Check sheet for the drawn part. Datum: minimum x, y, z corner. Units: mm. A direction names the side the tool comes from. Coordinates: 2 decimals unless noted, no trailing zeros. Order: outer loops, then holes, each group sorted by start corner. A loop starts at its lowest first (then second) coordinate and runs counter-clockwise, first axis right, second up. Notation, with made-up numbers: (81.25, 20) - (120.25, 20) arc R12 cw to (120.25, 28) - close; hole circle Ø1 at (75.5, -7). An arc over 180 degrees is marked (long way). One line per item, written item: value. Start each with the question number.
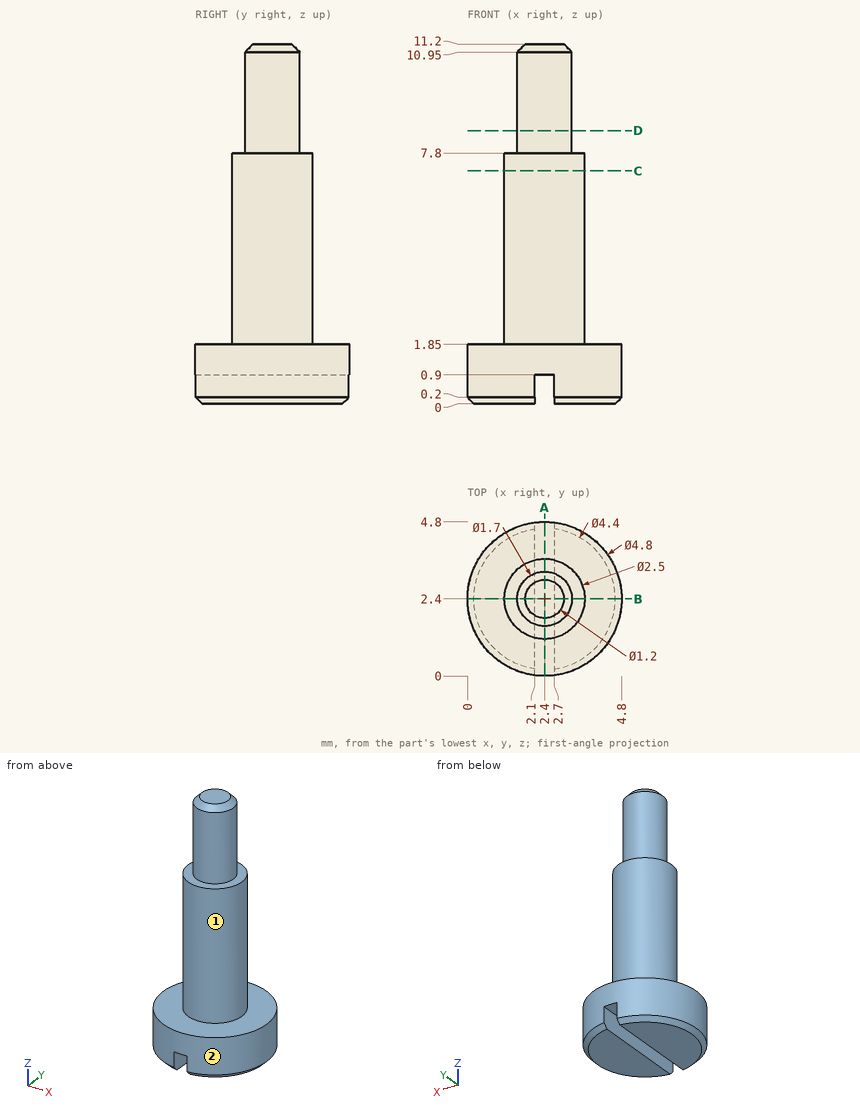
Q1. Cross-section at B-B, the plane y = 2.4. Enter the section's corners in (x, z).
Q2. Cross-section at D-D, the plane z = 8.5. Enter the section's corners in (x, y), and give its area (3 significant figures).
Q3. Cross-section at C-C, the plane z = 7.25. Enter the section's corners in (x, y).
Q4. Material ranges on probe 1 along Z at (x, y) = (1.5, 3.45); probe 2 along Z at (x, y) = (2.3, 2.3); probe 3 along X at (y, z) = (1.9, 2), recorded low to high.
Q5. Gauge pin test, flat ends, axial feed: P1, Ø0.5, axis at y = 3, z = 0, coming from the -X side; P2, Ø2, axis at x = 1, z = 7, coming from the -Y side; P3, Ø1.5, axis at x = 3, z = 3.5, coming from the +Y side. Record the tip position at first contact, or that the pin passes through.
Q6. Set-up check for the marked faces 1 and 2: record each of +Z, -Z, +X, -X, +Y, -Y from which the full face is reachable in a straight line by a thin tool's end or side.
Q7. Cross-section at A-A, the plane x = 2.4. Enter the section's corners in (y, z), and give its area (3 significant figures).
Check result:
1. outline: (0, 0.2) - (0.2, 0) - (2.1, 0) - (2.1, 0.9) - (2.7, 0.9) - (2.7, 0) - (4.6, 0) - (4.8, 0.2) - (4.8, 1.85) - (3.65, 1.85) - (3.65, 7.8) - (3.25, 7.8) - (3.25, 10.95) - (3, 11.2) - (1.8, 11.2) - (1.55, 10.95) - (1.55, 7.8) - (1.15, 7.8) - (1.15, 1.85) - (0, 1.85) - close
2. outline: circle Ø1.7 at (2.4, 2.4)
2. area: 2.27 mm2
3. outline: circle Ø2.5 at (2.4, 2.4)
4. probe 1: z = 0 to 1.85
4. probe 2: z = 0.9 to 11.2
4. probe 3: x = 1.25 to 3.55
5. P1: stops at x = 0.04
5. P2: stops at y = 1.22
5. P3: stops at y = 3.65
6. face 1: +Z
6. face 2: +Z, -Z
7. outline: (0, 0.9) - (4.8, 0.9) - (4.8, 1.85) - (3.65, 1.85) - (3.65, 7.8) - (3.25, 7.8) - (3.25, 10.95) - (3, 11.2) - (1.8, 11.2) - (1.55, 10.95) - (1.55, 7.8) - (1.15, 7.8) - (1.15, 1.85) - (0, 1.85) - close
7. area: 25.2 mm2
